Source: CAD feature listing. Evaluate the final solid. Frame: model axes, mm. Round coordinates to 2 decimals unless told otherwise and drop trailing zeros. Order: outer loops, then holes, each group sorted by start corner. A loop starts at its lowest first (then second) coordinate and runs counter-clockwise, first axis right, second up. Notation, with made-up numbers: (32.5, 45.5) -> (50.5, 45.5) arc R18 cw to (50.5, 50.5) -> close; hole circle Ø11 at (50, 21). An arc over 180 degrees is marked (long way). Answer as CSV lines item,"result".
from build123d import *

# Parameters (mm, degrees)
SKETCH_1_R          = 21.5
EXTRUDE_1_DEPTH     = 5.3
CUT_EXTRUDE_1_REACH = 32.864
SKETCH_2_R          = 1.35


with BuildPart() as part:
    # 草图1 → 凸台-拉伸1 (new body)
    with BuildSketch(Plane(origin=(0, 0, 0), x_dir=(1, 0, 0), z_dir=(0, 1, 0))):
        with Locations(Location((0, 0, 0), (0, 0, 270))):
            Circle(SKETCH_1_R)
    extrude(amount=EXTRUDE_1_DEPTH)

    # 草图2 → 切除-拉伸1 (cut, up to next)
    with BuildSketch(Plane(origin=(0, 5.3, 0), x_dir=(1, 0, 0), z_dir=(0, 1, 0)), mode=Mode.PRIVATE) as cut_extrude_1_sk1:
        with Locations(Location((-17.5, 0, 0), (0, 0, 270))):
            Circle(SKETCH_2_R)
    cut_extrude_1_tool1 = extrude(cut_extrude_1_sk1.sketch, amount=-CUT_EXTRUDE_1_REACH, mode=Mode.PRIVATE) & part.part
    # 草图2 → 切除-拉伸1 (cut, up to next)
    with BuildSketch(Plane(origin=(0, 5.3, 0), x_dir=(1, 0, 0), z_dir=(0, 1, 0)), mode=Mode.PRIVATE) as cut_extrude_1_sk2:
        with Locations(Location((0, 17.5, 0), (0, 0, 270))):
            Circle(SKETCH_2_R)
    cut_extrude_1_tool2 = extrude(cut_extrude_1_sk2.sketch, amount=-CUT_EXTRUDE_1_REACH, mode=Mode.PRIVATE) & part.part
    # 草图2 → 切除-拉伸1 (cut, up to next)
    with BuildSketch(Plane(origin=(0, 5.3, 0), x_dir=(1, 0, 0), z_dir=(0, 1, 0)), mode=Mode.PRIVATE) as cut_extrude_1_sk3:
        with Locations(Location((17.5, 0, 0), (0, 0, 270))):
            Circle(SKETCH_2_R)
    cut_extrude_1_tool3 = extrude(cut_extrude_1_sk3.sketch, amount=-CUT_EXTRUDE_1_REACH, mode=Mode.PRIVATE) & part.part
    # 草图2 → 切除-拉伸1 (cut, up to next)
    with BuildSketch(Plane(origin=(0, 5.3, 0), x_dir=(1, 0, 0), z_dir=(0, 1, 0)), mode=Mode.PRIVATE) as cut_extrude_1_sk4:
        with Locations(Location((0, -17.5, 0), (0, 0, 270))):
            Circle(SKETCH_2_R)
    cut_extrude_1_tool4 = extrude(cut_extrude_1_sk4.sketch, amount=-CUT_EXTRUDE_1_REACH, mode=Mode.PRIVATE) & part.part
    add(cut_extrude_1_tool1.solids().sort_by_distance((-17.5, 5.3, 0))[0], mode=Mode.SUBTRACT)
    add(cut_extrude_1_tool2.solids().sort_by_distance((0, 5.3, -17.5))[0], mode=Mode.SUBTRACT)
    add(cut_extrude_1_tool3.solids().sort_by_distance((17.5, 5.3, 0))[0], mode=Mode.SUBTRACT)
    add(cut_extrude_1_tool4.solids().sort_by_distance((0, 5.3, 17.5))[0], mode=Mode.SUBTRACT)


solid = part.part
1. Section query B-B on x = 17.5. Return loops of the section in (y, z), and give its area (3 significant figures).
Results below:
outline,"(0, -12.49) -> (5.3, -12.49) -> (5.3, -1.35) -> (0, -1.35) -> close; (0, 1.35) -> (5.3, 1.35) -> (5.3, 12.49) -> (0, 12.49) -> close"
area,"118 mm2"
2. Line query: L1, parallel to X at y = 3.1, z = 0; L2, parallel to X at y = 5, z = -17; L3, parallel to X at y = 2.35, z = 17.5. Output: solid intervals per line, ascending. Write a range as [from, to].
Results below:
L1,"[-21.5, -18.85], [-16.15, 16.15], [18.85, 21.5]"
L2,"[-13.16, -1.25], [1.25, 13.16]"
L3,"[-12.49, -1.35], [1.35, 12.49]"
3. Section query A-A on z = -17.5. Return loops of the section in (x, y), and give its area (3 significant figures).
Results below:
outline,"(-12.49, 0) -> (-1.35, 0) -> (-1.35, 5.3) -> (-12.49, 5.3) -> close; (1.35, 0) -> (12.49, 0) -> (12.49, 5.3) -> (1.35, 5.3) -> close"
area,"118 mm2"
4. Mould query, pull axis Z, two halves, no side actions, for faces 1 (the cylindrical face through (14.531, 2.613, -15.846)), 2 (the cylindrical face through (16.3, 2.69, 0.62)), 3 (the cylindrical face through (-16.362, 2.687, 0.726)), 4 (the flat face through (0, 5.3, 0)). Classes: released by +Z, released by -Z, zero draft, split by the parting line, or undercut.
Results below:
face 1,"split by the parting line"
face 2,"undercut"
face 3,"undercut"
face 4,"zero draft"
5. Pin query (flat end, axial travel): pin 1 (1 mm diameter, centred on y = 0.5, z = 7, fed in from +X); pin 2 (3 mm diameter, centred on x = 0, z = 17.5, fed in from +Y); pin 3 (1.5 mm diameter, centred on y = 4, z = -5, fed in from -X); pin 4 (1 mm diameter, centred on y = 4.5, z = -17, fed in from -X). Return the tip coordinate at first contact, or that it passes through.
Results below:
pin 1,"x = 20.49"
pin 2,"y = 5.3"
pin 3,"x = -21.08"
pin 4,"x = -13.78"
6. Section query D-D on z = 0. Return loops of the section in (x, y), and give its area (3 significant figures).
Results below:
outline,"(-21.5, 0) -> (-18.85, 0) -> (-18.85, 5.3) -> (-21.5, 5.3) -> close; (-16.15, 0) -> (16.15, 0) -> (16.15, 5.3) -> (-16.15, 5.3) -> close; (18.85, 0) -> (21.5, 0) -> (21.5, 5.3) -> (18.85, 5.3) -> close"
area,"199 mm2"
7. Section query C-C on x = 0. Return loops of the section in (y, z), and give its area (3 significant figures).
Results below:
outline,"(0, -21.5) -> (5.3, -21.5) -> (5.3, -18.85) -> (0, -18.85) -> close; (0, -16.15) -> (5.3, -16.15) -> (5.3, 16.15) -> (0, 16.15) -> close; (0, 18.85) -> (5.3, 18.85) -> (5.3, 21.5) -> (0, 21.5) -> close"
area,"199 mm2"
